Check sheet for the modelled part. Datum: model origin and axes. Units: mm. Face numbers are marked on the shaded views. A direction names the side the tool comes from. Give positions to 0.01 mm unless a question says otherwise; leave off trailing zeros. Write each loop counter-clockwise with the first axis right and the second up, starting at its lowest first coordinate (ties: lowest second). Pieces come first, ordered by that corner, then holes. Notation, with made-up numbers: (80, 1) -> (98, 1) arc R25 cw to (98, 25) -> close; hole circle Ø5 at (-24, 10.5). An arc over 180 degrees is marked (long way). Write each question's results on one line, items separated by ' | '. Start each with the question number.
```python
from build123d import *

# Parameters (mm, degrees)
SKETCH1_R                = 15
SKETCH1_R_2              = 13
BOSS_EXTRUDE2_DEPTH      = 12.6
BOSS_EXTRUDE3_DEPTH      = 3
BOSS_EXTRUDE3_DEPTH_BACK = 1


with BuildPart() as part:
    # Sketch1 → Boss-Extrude2 (new body)
    with BuildSketch(Plane(origin=(0, 0, 0), x_dir=(1, 0, 0), z_dir=(0, 1, 0))):
        with Locations((2.543609681, -2.543609681)):
            Circle(SKETCH1_R)
        with Locations((2.543609681, -2.543609681)):
            Circle(SKETCH1_R_2, mode=Mode.SUBTRACT)
    extrude(amount=BOSS_EXTRUDE2_DEPTH)

    # Sketch3 → Boss-Extrude3 (add, two sides)
    with BuildSketch(Plane(origin=(17.543609681, 0, 0), x_dir=(0, 0, -1), z_dir=(1, 0, 0))) as boss_extrude3_sk:
        Polygon((-5.043609681, 6.3), (-5.043609681, 8.8), (-0.043609681, 8.8), (-0.043609681, 6.3), (-0.043609681, 3.8), (-5.043609681, 3.8), align=None)
    extrude(amount=BOSS_EXTRUDE3_DEPTH)
    extrude(boss_extrude3_sk.sketch, amount=-BOSS_EXTRUDE3_DEPTH_BACK)


solid = part.part
```
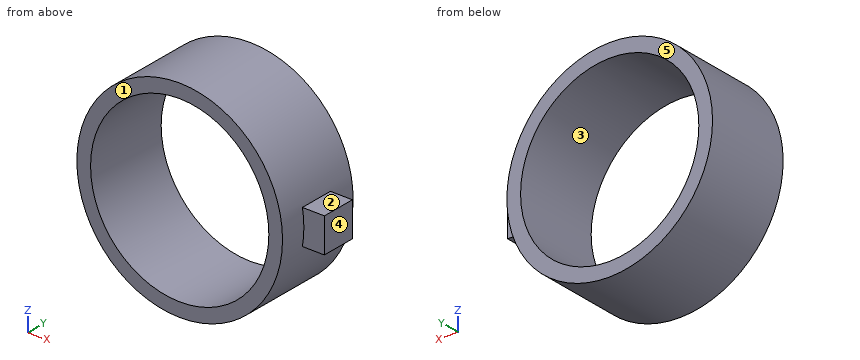
Item 1: Section check D-D on y = 10.25. Record the boundary of the cut face in (x, z), then the cut area to 3 significant figures.
Item 2: Mould release check, pull along X, two halves, no side actions. Record for the marked faces 3, 4 and 5: pulls with the +X half, pulls with the -X half, needs draft (parallel to the pull), parting line crosses it, or undercut.
Item 3: Section check C-C on y = 5.5. Record the boundary of the cut face in (x, z), then the cut area to 3 significant figures.
Item 4: Set-up check for the marked faces 1 and 2: record each of +Z, -Z, +X, -X, +Y, -Y from which the full face is reachable in a straight line by a thin tool's end or side.
Item 5: Section check B-B on z = 8.75. Record the boundary of the cut face in (x, y).
Item 6: Depth check by flat-ended pin: pin 1 Ø1.5 at (y, z) = (5.5, -2) entering from -X; pin 2 Ø1.5 at (y, z) = (2.5, 11) entering from +X; pin 3 Ø4 at (x, z) = (-3, 13.5) entering from -Y; pin 4 Ø1 at (x, y) = (18, 5.5) entering from +Z. Enter the tip coordinate at first touch or a pass-through.
Item 7: Section check A-A on x = 4. Record the boundary of the cut face in (y, z), then the cut area to 3 significant figures.
Item 8: Thickness scan on probe 1 along Z at (x, y) = (-6.5, 5); probe 2 along X at (y, z) = (8, 10.75); probe 3 along Z at (x, y) = (-7, 9.25). Record the ranges inside material, lowest first. Write a range as from..to.
Check sheet entries:
1) outline: circle Ø30 at (2.54, 2.54); hole circle Ø26 at (2.54, 2.54) | area: 176 mm^2
2) face 3: undercut | face 4: pulls with the +X half | face 5: needs draft
3) outline: (17.33, 0.04) -> (20.54, 0.04) -> (20.54, 5.04) -> (17.33, 5.04) arc R15 ccw (long way) to start; hole circle Ø26 at (2.54, 2.54) | area: 191 mm^2
4) face 1: +Z, -Z, +X, -X, -Y | face 2: +Z, +X, +Y, -Y
5) outline: (-11.11, 0) -> (-8.88, 0) -> (-8.88, 12.6) -> (-11.11, 12.6) -> close; (13.97, 0) -> (16.2, 0) -> (16.2, 12.6) -> (13.97, 12.6) -> close
6) pin 1: stops at x = -11.97 | pin 2: stops at x = 15.41 | pin 3: stops at y = 0 | pin 4: stops at z = 5.04
7) outline: (0, -12.39) -> (12.6, -12.39) -> (12.6, -10.37) -> (0, -10.37) -> close; (0, 15.46) -> (12.6, 15.46) -> (12.6, 17.47) -> (0, 17.47) -> close | area: 50.7 mm^2
8) probe 1: z = -9.42..-6.8, 11.88..14.51 | probe 2: x = -10.01..-7.54, 12.63..15.1 | probe 3: z = -9.03..-6.28, 11.37..14.12
